Solid Edge part; units mm, degrees
sketch "Sketch1" plane through (0, 0, 0) normal (0, -1, 0) x (1, 0, 0)
  line L0 (20, 7.5) -> (-20, 7.5)
  line L1 (-20, 7.5) -> (-20, -7.5)
  line L2 (-20, -7.5) -> (20, -7.5)
  line L3 (20, -7.5) -> (20, 7.5)
extrude "Protrusion1" add sketch "Sketch1" against normal blind 190
sketch "Sketch2" plane through (0, 75, -7.5) normal (0, 0, -1) x (0, 1, 0)
  line L0 (20, 20) -> (-7.1309, -20)
  line L1 (-7.1309, -20) -> (115, -20)
  line L2 (115, -20) -> (115, 20)
  line L3 (115, 20) -> (20, 20)
extrude "VaciadoExtruido_1" cut sketch "Sketch2" against normal blind 10
fillet "Redondeo_1" radius 20 4 edges at (20, 190, 5) (-20, 190, 5) (20, 0, 0) (-20, 0, 0)
sketch "Sketch3" plane through (0, 75, 7.5) normal (0, 0, 1) x (0, 1, 0)
  circle A0 centre (-55, 0) radius 9.5
extrude "VaciadoExtruido_2" cut sketch "Sketch3" against normal blind 37.5377
sketch "Sketch4" plane through (0, 75, 7.5) normal (0, 0, 1) x (0, 1, 0)
  circle A0 centre (95, 0) radius 9.5
extrude "VaciadoExtruido_3" cut sketch "Sketch4" against normal blind 32.4692
sketch "Sketch5" plane through (0, 95, 7.5) normal (0, 0, 1) x (0, -1, 0)
  line L0 (13.5655, 14) -> (35.5598, 14)
  line L1 (35.5598, -14) -> (35.5598, 14)
  line L2 (13.5655, 14) -> (35.5598, -14)
  line L3 (40.5598, 14) -> (40.5598, -14)
  line L4 (62.5498, 14) -> (40.5598, -14)
  line L5 (40.5598, 14) -> (62.5498, 14)
extrude "Cutout1" cut sketch "Sketch5" against normal blind 38.4793
mirror "Mirror1" about plane through (0, 95, 7.5) normal (0, -1, 0) of "Cutout1"
sketch "Sketch6" plane through (0, 95, 7.5) normal (0, 0, 1) x (0, 1, 0)
  line L0 (3.6809, -14) -> (25.6752, 14)
  line L1 (25.6752, 14) -> (-18.3134, 14)
  line L2 (-18.3134, 14) -> (3.6809, -14)
extrude "VaciadoExtruido_9" cut sketch "Sketch6" against normal blind 77.1311
The listing builds one solid part. Answer for the finished solid, in the listing's coordinates (mm). A direction names the side the tool comes from. Round coordinates to 2 decimals unless told otherwise and drop trailing zeros. Write each loop counter-clockwise with the first axis right and the second up, starting at its lowest first coordinate (ties: lowest second). Pieces come first, ordered by that corner, then holes. Notation, with made-up numbers: M 6.25,73.5 L 44.25,73.5 A33 cw 44.25,104.5 Z; hole C 61.25,66.5 d2. An arc over 180 degrees is marked long. Write each question's results on one line, items separated by ' | '. Start each with the question number.
(1) Determine the mould class of faces 1 (the cylindrical face through (14.297, 183.986, 5.035)), 2 (the flat face through (0.28, 81.624, -2.57)), 3 (the flat face through (14, 44, 0)), 4 (the flat face through (14, 147, 5)) for opening direction X: +X half, -X half, draft (parallel to the pull), parting line (faces both ways), or undercut.
(2) Each of these flat-tipped pins is pushed along its axis until it touches: P1, Ø1.5, axis at y = 112.5, z = 1.5, coming from the -X side; P2, Ø7.5, axis at x = 4.5, z = -3.5, coming from the -Y side; P3, Ø8, axis at x = 13.5, z = -1, coming from the -Y side; P4, Ø2, axis at x = 6.5, z = -1.5, coming from the -Y side. Where does it stop, or does it pass through?
(3) The part is cut by section A-A, the plane z = -2. Give the number of separate pieces and of enclosed holes in the cut face, and give its area (3 significant figures).
(4) For faces 5 (the flat face through (-20, 77, 3)), 6 (the flat face through (-0.2, 119.72, 5.04)), 7 (the flat face through (-9, 143, 2.5)), determine the directions among +Z, -Z, +X, -X, +Y, -Y from which every point of the face is accessible in a straight line to the end or side of a thin tool.
(5) Find the intervals of material crossed by line 1 (X direction, y = 20, z = 3.5); line 2 (Y direction, x = 0, z = -1.25); line 3 (Y direction, x = 12, z = 3.5), in increasing order.
(6) The part is cut by section C-C, the plane y = 39. Write down the section's boundary in (x, z), and give its area (3 significant figures).
Worked answers:
1) face 1: +X half | face 2: -X half | face 3: undercut | face 4: undercut
2) P1: passes through | P2: stops at y = 0.01 | P3: stops at y = 2.4 | P4: stops at y = 0.77
3) separate pieces: 1 | enclosed holes: 3 | area: 2,190 mm²
4) face 5: +Z, -Z, -X, +Y, -Y | face 6: +Z, -Z | face 7: -Z, -X, +Y
5) line 1: x = -20 to -9.5, 9.5 to 20 | line 2: y = 0 to 10.5, 29.5 to 43.45, 54.44 to 59.44, 70.44 to 81.43 | line 3: y = 4 to 34.02, 54.44 to 59.44, 79.86 to 97.11, 100.25 to 110.14, 130.56 to 135.56, 155.98 to 186
6) outline: M -20,-7.5 L 5.66,-7.5 L 5.66,7.5 L -20,7.5 Z; M 14,-7.5 L 20,-7.5 L 20,7.5 L 14,7.5 Z | area: 475 mm²
